The listing builds one solid part. Answer for the finished solid, in the listing's coordinates (mm). Coordinates: 2 decimals unless noted, no trailing zeros. Order: outer loops, then holes, each group sorted by start corner. A loop starts at its lowest first (then second) coordinate and runs counter-clockwise, first axis right, second up. Notation, with made-up numbers: (14.25, -12) -> (47.25, -12) arc R11 ccw to (47.25, 8) -> close; hole circle Ø5 at (79, 18). An arc over 180 degrees is marked (long way). Return JSON: item names as keys, results as strings.
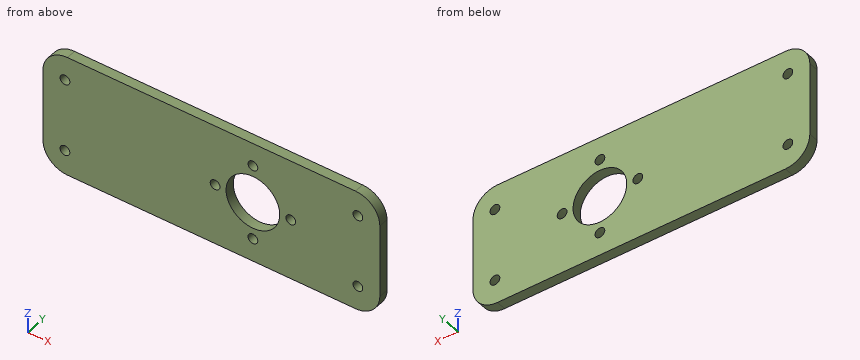
from build123d import *

# Parameters (mm, degrees)
SKETCH_1_W          = 143
SKETCH_1_H          = 50
SKETCH_1_R          = 2
SKETCH_1_R_2        = 11
EXTRUDE_1_DEPTH     = 4
SKETCH_4_W          = 5
SKETCH_4_H          = 50
CUT_EXTRUDE_3_DEPTH = 95.45633912
SKETCH_5_R          = 2
CUT_EXTRUDE_4_DEPTH = 90.649316785
FILLET_1_R          = 10


with BuildPart() as part:
    # 草图1 → 凸台-拉伸1 (new body)
    with BuildSketch(Plane(origin=(0, 0, 0), x_dir=(1, 0, 0), z_dir=(0, 1, 0))):
        with Locations((-19.5, 0)):
            Rectangle(SKETCH_1_W, SKETCH_1_H)
        with Locations(Location((-15.5, 0, 0), (0, 0, 270))):
            Circle(SKETCH_1_R, mode=Mode.SUBTRACT)
        with Locations(Location((0, 15.5, 0), (0, 0, 270))):
            Circle(SKETCH_1_R, mode=Mode.SUBTRACT)
        with Locations(Location((0, -15.5, 0), (0, 0, 270))):
            Circle(SKETCH_1_R, mode=Mode.SUBTRACT)
        with Locations(Location((43, -15, 0), (0, 0, 270))):
            Circle(SKETCH_1_R, mode=Mode.SUBTRACT)
        with Locations(Location((43, 15, 0), (0, 0, 270))):
            Circle(SKETCH_1_R, mode=Mode.SUBTRACT)
        with Locations(Location((0, 0, 0), (0, 0, 270))):
            Circle(SKETCH_1_R_2, mode=Mode.SUBTRACT)
        with Locations(Location((15.5, 0, 0), (0, 0, 270))):
            Circle(SKETCH_1_R, mode=Mode.SUBTRACT)
    extrude(amount=EXTRUDE_1_DEPTH)

    # 草图4 → 切除-拉伸3 (cut, through all)
    with BuildSketch(Plane(origin=(0, 4, 0), x_dir=(1, 0, 0), z_dir=(0, 1, 0))):
        with Locations((-88.5, 0)):
            Rectangle(SKETCH_4_W, SKETCH_4_H)
    extrude(amount=-CUT_EXTRUDE_3_DEPTH, mode=Mode.SUBTRACT)

    # 草图5 → 切除-拉伸4 (cut, through all)
    with BuildSketch(Plane(origin=(0, 4, 0), x_dir=(1, 0, 0), z_dir=(0, 1, 0))):
        with Locations(Location((-77, 15, 0), (0, 0, 270))):
            Circle(SKETCH_5_R)
        with Locations(Location((-77, -15, 0), (0, 0, 270))):
            Circle(SKETCH_5_R)
    extrude(amount=-CUT_EXTRUDE_4_DEPTH, mode=Mode.SUBTRACT)

    # 圆角1
    fillet_1_edges = [part.edges().sort_by_distance(p)[0] for p in [
        (52, 2, -25),
        (52, 2, 25),
        (-86, 2, -25),
        (-86, 2, 25),
    ]]
    fillet(fillet_1_edges, radius=FILLET_1_R)


solid = part.part
1. This flat-tipped pin is pushed along its axis until it touches: pin 1 Ø3.5 at (x, z) = (43, 15) entering from -Y. Where does it stop, or does it pass through?
Answer block:
{"pin 1": "passes through"}
2. The part is cut by section C-C on z = -5.5. Give the vertices of the cut face in (x, y), and give its area (3 significant figures).
Answer block:
{"outline": "(-86, 0) -> (-9.53, 0) -> (-9.53, 4) -> (-86, 4) -> close; (9.53, 0) -> (52, 0) -> (52, 4) -> (9.53, 4) -> close", "area": "476 mm2"}
3. The part is cut by section B-B on x = 0. Give the vertices of the cut face in (y, z).
Answer block:
{"outline": "(0, -25) -> (4, -25) -> (4, -17.5) -> (0, -17.5) -> close; (0, -13.5) -> (4, -13.5) -> (4, -11) -> (0, -11) -> close; (0, 11) -> (4, 11) -> (4, 13.5) -> (0, 13.5) -> close; (0, 17.5) -> (4, 17.5) -> (4, 25) -> (0, 25) -> close"}
4. The part is cut by section A-A on y = 2.8. Give the number of separate pieces and of enclosed holes in the cut face, and give its area (3 significant figures).
Answer block:
{"separate pieces": "1", "enclosed holes": "9", "area": "6,330 mm2"}
5. Consider line 1 (X direction, y = 2.4, z = 0); line 2 (X direction, y = 0.75, z = -15.5); line 3 (X direction, y = 0.25, z = 10). Determine where each line is inside the solid, lowest interval first. Write a range as from..to.
Answer block:
{"line 1": "x = -86..-17.5, -13.5..-11, 11..13.5, 17.5..52", "line 2": "x = -85.99..-78.94, -75.06..-2, 2..41.06, 44.94..51.99", "line 3": "x = -86..-4.58, 4.58..52"}
6. The part is cut by section D-D on z = 21.5. Give the vertices of the cut face in (x, y).
Answer block:
{"outline": "(-83.6, 0) -> (49.6, 0) -> (49.6, 4) -> (-83.6, 4) -> close"}
